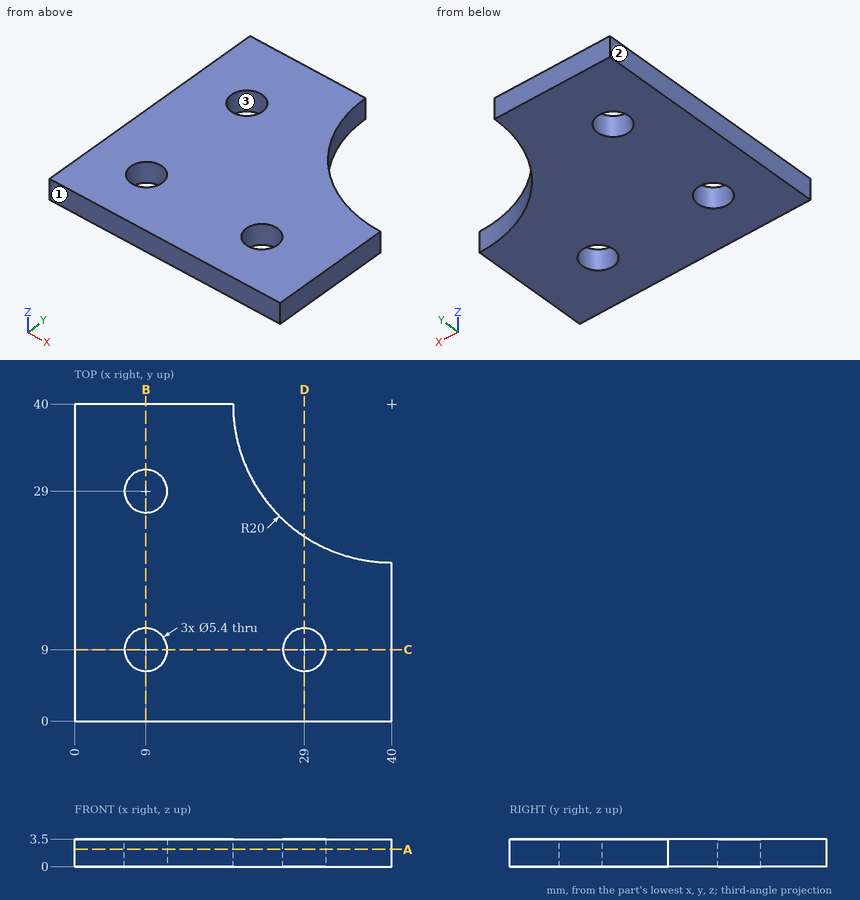
Answer from the drawing. Dimensions are ordinates in mm from the lowest x, y and z of the part. Round coordinates to 2 decimals unless told otherwise and drop trailing zeros. Loops run counter-clockwise (first coordinate to the right, second up) from the corner with the lowest first, then second, coordinate; pieces in that order, holes last. Notation, with made-up numbers: (-37, -19) - (7, -19) arc R20 ccw to (7, -2) - close; hole circle Ø7 at (-26.75, 22.5). An arc over 180 degrees is marked (long way). One line per item, written item: value.
Q1. Straight lines are drawn through the part: probe 1 along Y at (x, z) = (9, 1.5); probe 2 along Y at (x, z) = (8, 1.65); probe 3 along Y at (x, z) = (29, 0.95). For each, find the intervals that lie inside material, in ascending order.
Check values:
probe 1: 0 to 6.3, 11.7 to 26.3, 31.7 to 40
probe 2: 0 to 6.49, 11.51 to 26.49, 31.51 to 40
probe 3: 0 to 6.3, 11.7 to 23.3
Q2. Find section B-B on x = 9. Give the vertices of the cut face in (y, z), and give its area (3 significant figures).
Check values:
outline: (0, 0) - (6.3, 0) - (6.3, 3.5) - (0, 3.5) - close; (11.7, 0) - (26.3, 0) - (26.3, 3.5) - (11.7, 3.5) - close; (31.7, 0) - (40, 0) - (40, 3.5) - (31.7, 3.5) - close
area: 102 mm2
Q3. Find section A-A on z = 2.2. Give the vertices of the cut face in (x, y), and give its area (3 significant figures).
Check values:
outline: (0, 0) - (40, 0) - (40, 20) arc R20 cw to (20, 40) - (0, 40) - close; hole circle Ø5.4 at (9, 9); hole circle Ø5.4 at (9, 29); hole circle Ø5.4 at (29, 9)
area: 1,220 mm2
Q4. The mould has two halves that part along X. Classify the marked faces 1, 2 and 3: +X half, -X half, draft (parallel to the pull), parting line (faces both ways), or undercut.
Check values:
face 1: draft
face 2: -X half
face 3: undercut
Q5. Find section D-D on x = 29. Give the vertices of the cut face in (y, z).
Check values:
outline: (0, 0) - (6.3, 0) - (6.3, 3.5) - (0, 3.5) - close; (11.7, 0) - (23.3, 0) - (23.3, 3.5) - (11.7, 3.5) - close
Q6. Each of these flat-tipped pins is pushed along its axis until it touches: pin 1 Ø4 at (x, y) = (5.5, 20.5) entering from -Z; pin 2 Ø4.5 at (x, y) = (29, 9) entering from -Z. Where does it stop, or does it pass through?
Check values:
pin 1: z = 0
pin 2: through
